```python
from build123d import *

# Parameters (mm, degrees)
PAD_DEPTH            = 46
PAD_DEPTH_BACK       = 30
SKETCH009_R          = 8.650139
POCKET006_DEPTH      = 4.25
SKETCH011_R          = 1.5
POCKET008_DEPTH      = 9.501
POCKET008_DEPTH_BACK = 0.001
SKETCH010_R          = 8.650139
SKETCH010_R_2        = 3
POCKET007_DEPTH      = 5
SKETCH005_R          = 5.8
POCKET002_DEPTH      = 9.501
POCKET002_DEPTH_BACK = 0.001
SKETCH006_R          = 6.1
POCKET003_DEPTH      = 5.75
POCKET004_DEPTH      = 9.501
POCKET004_DEPTH_BACK = 0.001
SKETCH008_W          = 4
SKETCH008_H          = 12.2
POCKET005_DEPTH      = 5.75
POCKET009_DEPTH      = 9.501
POCKET009_DEPTH_BACK = 0.001
POCKET_DEPTH         = 2.751
SKETCH014_R          = 3.035
POCKET010_DEPTH      = 31.001
PAD001_DEPTH         = 9.5
SKETCH017_R          = 1.6
POCKET011_DEPTH      = 9.501
SKETCH018_W          = 100
SKETCH018_H          = 100
POCKET012_DEPTH      = 5.501
SKETCH020_R          = 8
SKETCH019_R          = 6
SKETCH021_R          = 8
POCKET013_DEPTH      = 5.501
SKETCH023_W          = 100
SKETCH023_H          = 16
SKETCH022_W          = 100
SKETCH022_H          = 12
SKETCH024_W          = 100
SKETCH024_H          = 16
SKETCH025_R          = 1.6
POCKET014_DEPTH      = 9.501
FILLET_R             = 3
FILLET001_R          = 2
FILLET002_R          = 0.43
FILLET003_R          = 3
POCKET015_DEPTH      = 4.5
CHAMFER_SIZE         = 1.14
SKETCH027_W          = 50
SKETCH027_H          = 0.5
POCKET016_DEPTH      = 4.25


with BuildPart() as part:
    # Sketch → Pad (new body, two sides)
    with BuildSketch(Plane.YZ) as pad_sk:
        Polygon((0, -9.5), (22, -9.5), (22, 0), (-22, 0), (-22, -9.5), align=None)
    extrude(amount=PAD_DEPTH)
    extrude(pad_sk.sketch, amount=-PAD_DEPTH_BACK)

    # Sketch009 → Pocket006 (cut, symmetric)
    with BuildSketch(Plane.XY):
        with Locations((5, -17.25)):
            Circle(SKETCH009_R)
        with Locations((5, 17.25)):
            Circle(SKETCH009_R)
    extrude(amount=POCKET006_DEPTH, both=True, mode=Mode.SUBTRACT)

    # Sketch011 → Pocket008 (cut, two sides)
    with BuildSketch(Plane.XY) as pocket008_sk:
        with Locations((5, 17.25)):
            Circle(SKETCH011_R)
        with Locations((5, -17.25)):
            Circle(SKETCH011_R)
    extrude(amount=-POCKET008_DEPTH, mode=Mode.SUBTRACT)
    extrude(pocket008_sk.sketch, amount=POCKET008_DEPTH_BACK, mode=Mode.SUBTRACT)

    # Sketch010 → Pocket007 (cut, symmetric)
    with BuildSketch(Plane.XY):
        with Locations((5, -17.25)):
            Circle(SKETCH010_R)
        with Locations((5, -17.25)):
            Circle(SKETCH010_R_2, mode=Mode.SUBTRACT)
        with Locations((5, 17.25)):
            Circle(SKETCH010_R)
        with Locations((5, 17.25)):
            Circle(SKETCH010_R_2, mode=Mode.SUBTRACT)
    extrude(amount=POCKET007_DEPTH, both=True, mode=Mode.SUBTRACT)

    # Sketch005 → Pocket002 (cut, two sides)
    with BuildSketch(Plane.XY) as pocket002_sk:
        with Locations((9, 0)):
            Circle(SKETCH005_R)
    extrude(amount=-POCKET002_DEPTH, mode=Mode.SUBTRACT)
    extrude(pocket002_sk.sketch, amount=POCKET002_DEPTH_BACK, mode=Mode.SUBTRACT)

    # Sketch006 → Pocket003 (cut)
    with BuildSketch(Plane.XY):
        with Locations((9, 0)):
            Circle(SKETCH006_R)
    extrude(amount=-POCKET003_DEPTH, mode=Mode.SUBTRACT)

    # Sketch007 → Pocket004 (cut, two sides)
    with BuildSketch(Plane.XY) as pocket004_sk:
        Polygon((9, 0), (11.086323, 5.732125), (11.220218, 6.1), (111.220218, 6.1), (111.220218, -6.1), (11.220218, -6.1), (11.086323, -5.732125), align=None)
    extrude(amount=-POCKET004_DEPTH, mode=Mode.SUBTRACT)
    extrude(pocket004_sk.sketch, amount=POCKET004_DEPTH_BACK, mode=Mode.SUBTRACT)

    # Sketch008 → Pocket005 (cut)
    with BuildSketch(Plane.XY):
        with Locations((11, 0)):
            Rectangle(SKETCH008_W, SKETCH008_H)
    extrude(amount=-POCKET005_DEPTH, mode=Mode.SUBTRACT)

    # Sketch012 → Pocket009 (cut, two sides)
    with BuildSketch(Plane.XY) as pocket009_sk:
        with BuildLine():
            ThreePointArc((31.8, 12.35), (30.2, 10.75), (31.8, 9.15))
            Line((31.8, 9.15), (36.2, 9.15))
            ThreePointArc((36.2, 9.15), (37.8, 10.75), (36.2, 12.35))
            Line((31.8, 12.35), (36.2, 12.35))
        make_face()
        with BuildLine():
            ThreePointArc((31.8, -9.15), (30.2, -10.75), (31.8, -12.35))
            Line((31.8, -12.35), (36.2, -12.35))
            ThreePointArc((36.2, -12.35), (37.8, -10.75), (36.2, -9.15))
            Line((31.8, -9.15), (36.2, -9.15))
        make_face()
    extrude(amount=-POCKET009_DEPTH, mode=Mode.SUBTRACT)
    extrude(pocket009_sk.sketch, amount=POCKET009_DEPTH_BACK, mode=Mode.SUBTRACT)

    # Sketch013 (on DatumPlane) → Pocket (cut, through all)
    with BuildSketch(Plane.XY.offset(-6.75)):
        with BuildLine():
            ThreePointArc((9, 6.1), (2.9, 0), (9, -6.1))
            Line((9, -6.1), (34, -6.1))
            Line((34, 6.1), (34, -6.1))
            Line((9, 6.1), (34, 6.1))
        make_face()
    extrude(amount=-POCKET_DEPTH, mode=Mode.SUBTRACT)

    # Sketch014 (on DatumPlane) → Pocket010 (cut, through all)
    with BuildSketch(Plane.YZ.offset(15)):
        with Locations((-16, 0)):
            Circle(SKETCH014_R)
        with Locations((16, 0)):
            Circle(SKETCH014_R)
    extrude(amount=POCKET010_DEPTH, mode=Mode.SUBTRACT)

    # Sketch016 → Pad001 (join)
    with BuildSketch(Plane.XY):
        Polygon((13, -22), (46, -22), (46, -24), (15.856296, -24), align=None)
        Polygon((13, 22), (46, 22), (46, 24), (15.856296, 24), align=None)
    extrude(amount=-PAD001_DEPTH)

    # Sketch017 → Pocket011 (cut, through all)
    with BuildSketch(Plane.XY):
        with Locations((26.25, -10.75)):
            Circle(SKETCH017_R)
        with Locations((26.25, -21.25)):
            Circle(SKETCH017_R)
        with Locations((41.75, -21.25)):
            Circle(SKETCH017_R)
        with Locations((41.75, -10.75)):
            Circle(SKETCH017_R)
        with Locations((26.25, 10.75)):
            Circle(SKETCH017_R)
        with Locations((41.75, 10.75)):
            Circle(SKETCH017_R)
        with Locations((26.25, 21.25)):
            Circle(SKETCH017_R)
        with Locations((41.75, 21.25)):
            Circle(SKETCH017_R)
        with Locations((17, -10)):
            Circle(SKETCH017_R)
        with Locations((17, 10)):
            Circle(SKETCH017_R)
        with Locations((2, -6)):
            Circle(SKETCH017_R)
        with Locations((2, 6)):
            Circle(SKETCH017_R)
    extrude(amount=-POCKET011_DEPTH, mode=Mode.SUBTRACT)

    # Sketch018 (on DatumPlane) → Pocket012 (cut, through all)
    with BuildSketch(Plane.XY.offset(-5.5)):
        with Locations((-51.1, 0)):
            Rectangle(SKETCH018_W, SKETCH018_H)
    extrude(amount=POCKET012_DEPTH, mode=Mode.SUBTRACT)

    # Sketch020 (on DatumPlane) → SubtractiveLoft section 0
    with BuildSketch(Plane.XY.offset(-5.5)):
        with Locations((-7, 0)):
            Circle(SKETCH020_R)
    # Sketch019 (on DatumPlane) → SubtractiveLoft section 1
    with BuildSketch(Plane.XY.offset(-7.5)):
        with Locations((-7, 0)):
            Circle(SKETCH019_R)
    # Sketch021 (on DatumPlane) → SubtractiveLoft section 2
    with BuildSketch(Plane.XY.offset(-9.5)):
        with Locations((-7, 0)):
            Circle(SKETCH021_R)
    loft(ruled=True, mode=Mode.SUBTRACT)

    # Sketch020 (on DatumPlane) → Pocket013 (cut, through all)
    with BuildSketch(Plane.XY.offset(-5.5)):
        with Locations((-7, 0)):
            Circle(SKETCH020_R)
    extrude(amount=POCKET013_DEPTH, mode=Mode.SUBTRACT)

    # Sketch023 (on DatumPlane) → SubtractiveLoft001 section 0
    with BuildSketch(Plane.XY.offset(-5.5)):
        with Locations((-57, 0)):
            Rectangle(SKETCH023_W, SKETCH023_H)
    # Sketch022 (on DatumPlane) → SubtractiveLoft001 section 1
    with BuildSketch(Plane.XY.offset(-7.5)):
        with Locations((-57, 0)):
            Rectangle(SKETCH022_W, SKETCH022_H)
    # Sketch024 (on DatumPlane) → SubtractiveLoft001 section 2
    with BuildSketch(Plane.XY.offset(-9.5)):
        with Locations((-57, 0)):
            Rectangle(SKETCH024_W, SKETCH024_H)
    loft(ruled=True, mode=Mode.SUBTRACT)

    # Sketch025 → Pocket014 (cut, through all)
    with BuildSketch(Plane.XY):
        with Locations((-24, -14)):
            Circle(SKETCH025_R)
        with Locations((-24, 14)):
            Circle(SKETCH025_R)
    extrude(amount=-POCKET014_DEPTH, mode=Mode.SUBTRACT)

    # Fillet
    fillet_edges = [part.edges().sort_by_distance(p)[0] for p in [
        (-30, -22, -7.5),
        (-30, 22, -7.5),
        (-30, 7, -8.5),
        (-30, 7, -6.5),
        (-30, -7, -6.5),
        (-30, -7, -8.5),
    ]]
    fillet(fillet_edges, radius=FILLET_R)

    # Fillet001
    fillet001_edges = [part.edges().sort_by_distance(p)[0] for p in [
        (-1.1, -11.1169, -2.125),
        (-1.1, 11.1169, -2.125),
    ]]
    fillet(fillet001_edges, radius=FILLET001_R)

    # Fillet002
    fillet002_edges = [part.edges().sort_by_distance(p)[0] for p in [
        (12.229275, -22, -2.125),
        (12.229275, 22, -2.125),
    ]]
    fillet(fillet002_edges, radius=FILLET002_R)

    # Fillet003
    fillet003_edges = [part.edges().sort_by_distance(p)[0] for p in [
        (-1.1, -22, -5.25),
        (-1.1, 22, -5.25),
    ]]
    fillet(fillet003_edges, radius=FILLET003_R)

    # Sketch026 (on DatumPlane) → Pocket015 (cut)
    with BuildSketch(Plane.XY.offset(-9.5)):
        with BuildLine():
            ThreePointArc((29, 7.25), (21.75, 0), (29, -7.25))
            Line((29, -7.25), (49, -7.25))
            Line((49, 7.25), (49, -7.25))
            Line((29, 7.25), (49, 7.25))
        make_face()
    extrude(amount=POCKET015_DEPTH, mode=Mode.SUBTRACT)

    # Chamfer
    chamfer_edges = [part.edges().sort_by_distance(p)[0] for p in [
        (35.540887, 6.1, -5),
        (35.540887, -6.1, -5),
    ]]
    chamfer(chamfer_edges, length=CHAMFER_SIZE)

    # Sketch027 → Pocket016 (cut, symmetric)
    with BuildSketch(Plane.XY):
        with Locations((21, -23.75)):
            Rectangle(SKETCH027_W, SKETCH027_H)
        with Locations((21, 23.75)):
            Rectangle(SKETCH027_W, SKETCH027_H)
    extrude(amount=POCKET016_DEPTH, both=True, mode=Mode.SUBTRACT)


solid = part.part
```
The listing builds one solid part. Answer for the finished solid, in the listing's coordinates (mm). A direction names the side the tool comes from. Give positions to 0.01 mm unless a question says otherwise; leave off trailing zeros. Order: outer loops, then holes, each group sorted by start corner. A loop starts at its lowest first (then second) coordinate and runs counter-clockwise, first axis right, second up. Notation, with made-up numbers: M 15,21.5 L 57,21.5 A9 ccw 57,28.5 Z; hole C 3.5,59 d7. An arc over 180 degrees is marked long. Put each result on its own line as item: value. Start each with the question number.
Item 1: The part is cut by section D-D, the plane y = 0. Determine the outline of the cut face in (x, z), and give its area (4 significant figures).
Item 2: The part is cut by section A-A, the plane x = -14. Determine the outline of the cut face in (y, z), and give its area (3 significant figures).
Item 3: The part is cut by section C-C, the plane y = 17.25. Determine the outline of the cut face in (x, z).
Item 4: The part is cut by section B-B, the plane x = 33.5. State how many separate pieces and enclosed holes the cut face has, and give its area (3 significant figures).
Item 5: Find the intervals of material crossed by line 1 along Y through (x, z) = (17, -5.25); line 2 along Y through (x, z) = (41.75, -3.5); line 3 along Y through (x, z) = (17, -2), in increasing order.
Item 6: For a pull along X with two mould halves and no side action, classify faces 1 (the face through (-17.1, -7, -6.5)), 2 (the face through (8, 15, -5)), 3 (the face through (46, -15, -5)) as +X half, -X half, draft (parallel to the pull), parting line (faces both ways), or undercut.
Item 7: Which of the six approach directions +Z, -Z, +X, -X, +Y, -Y give full straight-line access (tool end or side, diameter ignored) to faces 4 (the face through (37, 7.25, -7)), 5 (the face through (30, -23.5, -2)), 6 (the face through (6, 19, -4.25)), 7 (the face through (8, -15, -5)), 8 (the face through (-16.9, 7, -8.5))?
Item 8: Flat-ended cylindrical pins translate along their axes: P1, Ø2, axis at x = 34, z = -3, coming from the +Y side; P2, Ø1.5, axis at y = 3.5, z = -1.5, coming from the -X side; P3, Ø1, axis at y = -3, z = -1.5, coming from the +X side; P4, Ø3, axis at x = 2, y = 6, coming from the +Z side. Find the tip coordinate at first contact, or state that the pin passes through.
Answer key:
1. outline: M -1,-7.5 L 1,-9.5 L 2.9,-9.5 L 2.9,-6.75 L 3.2,-6.75 L 3.2,-5.75 L 2.9,-5.75 L 2.9,0 L 1,0 L 1,-5.5 Z
1. area: 22.35 mm²
2. outline: M -22,-9.5 L -8,-9.5 L -6,-7.5 L -8,-5.5 L -22,-5.5 Z; M 6,-7.5 L 8,-9.5 L 22,-9.5 L 22,-5.5 L 8,-5.5 Z
2. area: 120 mm²
3. outline: M -30,-9.5 L 3.5,-9.5 L 3.5,-4.25 L 2,-4.25 L 2,-5 L -1.1,-5 L -1.1,-5.5 L -30,-5.5 Z; M 6.5,-9.5 L 46,-9.5 L 46,-2.77 L 15,-2.77 L 15,0 L 13.65,0 L 13.65,-5 L 8,-5 L 8,-4.25 L 6.5,-4.25 Z
4. separate pieces: 4
4. enclosed holes: 0
4. area: 234 mm²
5. line 1: y = -24 to -11.6, -8.4 to -6.1, 6.1 to 8.4, 11.6 to 24
5. line 2: y = -23.5 to -22.85, -19.65 to -12.35, -9.15 to -6.1, 6.1 to 9.15, 12.35 to 19.65, 22.85 to 23.5
5. line 3: y = -23.5 to -18.28, -13.72 to -11.6, -8.4 to -6.1, 6.1 to 8.4, 11.6 to 13.72, 18.28 to 23.5
6. face 1: draft
6. face 2: undercut
6. face 3: +X half
7. face 4: -Z, +X
7. face 5: +Z, +X, -X, -Y
7. face 6: +Z, -X, +Y
7. face 7: +Z
7. face 8: -Z, -X
8. P1: stops at y = 23.5
8. P2: stops at x = -0.22
8. P3: stops at x = 4
8. P4: passes through
